The model under review builds one solid part; all positions refer to its coordinate system, in mm. A direction names the side the tool comes from. Give positions to 0.01 mm unless a question says otherwise; leave off trailing zeros. Loops run counter-clockwise (first coordinate to the right, second up) from the corner with the lowest first, then second, coordinate; pieces in that order, holes last. Notation, with made-up numbers: M 85.5,22 L 120.5,22 A22 ccw 120.5,52 Z; hole C 36.5,30 d8. An arc over 180 degrees is marked long. Put each result on its own line as item: value. Start each with the question number.
```python
from build123d import *

# Parameters (mm, degrees)
BOX_W           = 50
BOX_H           = 40
BOX_DEPTH       = 30
POCKET_DEPTH    = 40.001
POCKET001_DEPTH = 5
POCKET002_DEPTH = 5


with BuildPart() as part:
    # Box → Box (new body)
    with BuildSketch(Plane.XY):
        with Locations((25, 20)):
            Rectangle(BOX_W, BOX_H)
    extrude(amount=BOX_DEPTH)

    # Sketch → Pocket (cut, through all)
    with BuildSketch(Plane.XZ):
        Polygon((17, 0), (5, 15), (45, 15), (33, 0), align=None)
    extrude(amount=-POCKET_DEPTH, mode=Mode.SUBTRACT)

    # Sketch001 → Pocket001 (cut)
    with BuildSketch(Plane.XY.offset(30)):
        Polygon((50, 0), (24, 0), (50, 21), align=None)
    extrude(amount=-POCKET001_DEPTH, mode=Mode.SUBTRACT)

    # Sketch003 → Pocket002 (cut)
    with BuildSketch(Plane.XY.offset(30)):
        Polygon((19, -0.009107), (14, -0.009107), (50.194458, 31), (50.194458, 26), align=None)
    extrude(amount=-POCKET002_DEPTH, mode=Mode.SUBTRACT)


solid = part.part
```
Item 1: Consider section D-D, the plane x = 29. Write out the cut boundary in (y, z), plus the area to 3 significant figures.
Item 2: Tool access review of faces 5 (the flat face through (25, 20, 15)), 6 (the flat face through (35, 15, 25)), 7 (the flat face through (43, 6, 25)): name each direction out of +Z, -Z, +X, -X, +Y, -Y from which nothing blocks a thin tool from reaching the whole face with its end or side.
Item 3: Draft analysis for pull direction Z (two halves, no side actions). For faces 1 (the flat face through (25, 0, 18)), 2 (the flat face through (11.08, 19.72, 7.4)), 3 (the flat face through (39.08, 19.72, 7.6)), 4 (the flat face through (41, 20, 0)), state which applies: +Z half, -Z half, draft (parallel to the pull), parting line (faces both ways), or undercut.
Item 4: Consider section C-C, the plane y = 32. Write out the cut boundary in (x, z).
Item 5: Consider section A-A, the plane z = 10. Write out the cut boundary in (x, y).
Item 6: To check wall thickness, follow L1, parallel to X at y = 11.5, z = 28.5; L2, parallel to Z at x = 5.5, y = 12 (3 decimals); L3, parallel to X at y = 13, z = 26. State the ranges of each line that lie inside material, in increasing order. Write a range as [from, to].
Item 7: Consider section B-B, the plane x = 9. Write out the cut boundary in (y, z), plus the area to 3 significant figures.
Report:
1. outline: M 0,15 L 40,15 L 40,30 L 12.84,30 L 12.84,25 L 8.33,25 L 8.33,30 L 4.04,30 L 4.04,25 L 0,25 Z
1. area: 557 mm²
2. face 5: +Y, -Y
2. face 6: +Z
2. face 7: +Z, +X, -Y
3. face 1: draft
3. face 2: undercut
3. face 3: undercut
3. face 4: -Z half
4. outline: M 0,0 L 17,0 L 5,15 L 45,15 L 33,0 L 50,0 L 50,30 L 0,30 Z
5. outline: M 0,0 L 9,0 L 9,40 L 0,40 Z; M 41,0 L 50,0 L 50,40 L 41,40 Z
6. L1: [0, 27.43], [32.8, 38.24]
6. L2: [0, 14.375], [15, 30]
6. L3: [0, 29.18], [34.6, 40.1]
7. outline: M 0,0 L 40,0 L 40,10 L 0,10 Z; M 0,15 L 40,15 L 40,30 L 0,30 Z
7. area: 1,000 mm²
